The listing builds one solid part. Answer for the finished solid, in the listing's coordinates (mm). Face numbers are marked on the shaded views. A direction names the side the tool comes from. Give positions to 0.01 mm unless a question says otherwise; leave off trailing zeros. Order: outer loops, then holes, each group sorted by start corner. A loop starts at its lowest first (then second) coordinate and runs counter-clockwise, first axis right, second up. Notation, with made-up numbers: (87.5, -12) - (114.5, -12) arc R14 cw to (114.5, 10) - close; hole circle Ø7 at (-32.75, 1). An arc over 180 degrees is marked (long way). Answer as CSV lines item,"result". Start each with the question number.
1. Section A-A on z = 1.5 is taken. Give the vertices of the cut face in (x, y) (3 decimals), and give its area (3 significant figures).
2. Which of the six approach directions +Z, -Z, +X, -X, +Y, -Y give full straight-line access (tool end or side, diameter ignored) to the marked faces 1, 2 and 3?
3. Section C-C on y = -13.9 is taken. Give the vertices of the cut face in (x, z) (3 decimals), and give its area (3 significant figures).
4. Determine the mould class of the marked faces 4, 5 and 6 for opening direction Z: +Z half, -Z half, draft (parallel to the pull), parting line (faces both ways), or undercut.
5. Section D-D on z = -1.25 is taken. Give the vertices of the cut face in (x, y) (3 decimals).
6. Flat-ended cylindrical pins translate along their axes: pin 1 (0.6 mm diameter, centred on x = -8.5, z = -7.5, fed in from +Y); pin 2 (1.6 mm diameter, centred on x = -9, y = 1, fed in from -Z); pin 3 (1.6 mm diameter, centred on x = 0, y = -13.9, fed in from +Z); pin 4 (4 mm diameter, centred on x = 0, y = 13.9, fed in from -Z). Find the tip coordinate at first contact, or state that the pin passes through.
7. Section B-B on x = 4 is taken. Give the vertices of the cut face in (y, z), and give its area (3 significant figures).
8. Consider line 1 along Y through (x, z) = (0, 4.3); line 2 along Z through (x, y) = (-4.15, -12.1) (3 decimals); line 3 along Y through (x, z) = (0, -3.25). Determine where each line is inside the solid, lowest interval first. Write a range as [from, to].
Autodesk Inventor part; units mm, degrees
ref_plane "Work Plane1" through (-1.325, -11.4, 0) normal (-1, 0, 0) x (0, 0, 1)
ref_plane "Work Plane3" through (0, -16.6, 5) normal (-1, 0, 0) x (0, 0, 1)
ref_plane "YZ Plane" through (0, 0, 0) normal (1, 0, 0) x (0, 1, 0)
sketch "Sketch1" plane through (0, 0, 0) normal (0, 0, 1) x (1, 0, 0)
  line L0 (-9.975, 16.6) -> (9.975, 16.6)
  line L1 (9.975, 16.6) -> (9.975, -16.6)
  line L2 (9.975, -16.6) -> (-9.975, -16.6)
  line L3 (-9.975, -16.6) -> (-9.975, 16.6)
  line L4 (0, 0) -> (0, 11.4) construction
  line L5 (0, 0) -> (15.5803, 0) construction
  line L6 (-6.15, 11.4) -> (6.15, 11.4)
  line L7 (6.15, 11.4) -> (6.15, -11.4)
  line L8 (6.15, -11.4) -> (-6.15, -11.4)
  line L9 (-6.15, -11.4) -> (-6.15, 11.4)
  circle A0 centre (0, 13.9) radius 1.3
  circle A1 centre (0, -13.9) radius 1.3
  line L10 (-15.0861, 0) -> (20.6914, 0)
  line L11 (9.975, -16.6) -> (-9.975, -16.6)
  line L12 (-9.975, -16.6) -> (-9.975, -11.4)
  line L13 (-9.975, -11.4) -> (9.975, -11.4)
  line L14 (9.975, -11.4) -> (9.975, -16.6)
  line L15 (0, 11.4) -> (0, 13.9) construction
  point P0 (0, 16.6)
  dimension "d0" = 2.6
  dimension "d1" = 27.8
  dimension "d4" = 12.3
  dimension "d5" = 2.5
  dimension "d6" = 2.5
  dimension "d7" = 22.8
  dimension "d11" = 2.7
  dimension "d12" = 2.7
  dimension "d14" = 3.825
extrude "Extrusion1" add sketch "Sketch1" along normal blind 5 contours L0 L1 L10 L7 L6 L9 L3 | L10 L9 L13 L3 | L1 L13 L7 L10 | L13 L8 L1 L2 L3
extrude "Extrusion2" add sketch "Sketch1" against normal blind 15.8 contours L13 L8 L1 L2 L3
sketch "Sketch2" plane through (-6.15, -11.4, 5) normal (0, 1, 0) x (1, 0, 0)
  circle A0 centre (10.3, 15.485) radius 1.05
  circle A1 centre (2, 15.485) radius 1.05
  line L0 (-3.825, 20.8) -> (16.125, 20.8)
  line L1 (-3.825, 5) -> (-3.825, 20.8)
  line L2 (2, 15.485) -> (10.3, 15.485) construction
  line L3 (10.3, 15.485) -> (6.15, 15.485) construction
  line L4 (6.15, 15.485) -> (6.15, 20.8) construction
  point P0 (6.15, 5)
  dimension "d19" = 2.1
  dimension "d20" = 0
  dimension "d21" = 5.315
  dimension "d22" = 8.3
extrude "Extrusion3" cut sketch "Sketch2" against normal blind 10
sketch "Sketch3" plane through (-6.15, -11.4, 5) normal (0, 1, 0) x (1, 0, 0)
  circle A0 centre (10.3, 15.485) radius 1.05
  circle A1 centre (10.3, 15.485) radius 2.5
  circle A2 centre (2, 15.485) radius 1.05
  circle A3 centre (2, 15.485) radius 2.5
  point P0 (6.15, 5)
  dimension "d26" = 5
extrude "Extrusion4" cut sketch "Sketch3" against normal blind 2
sketch "Sketch4" plane through (9.975, -11.4, 0) normal (1, 0, 0) x (0, 0, -1)
  line L0 (0, 0) -> (15.8, 0)
  line L1 (0, 0) -> (0, 28)
  line L2 (15.8, 0) -> (0, 28)
  line L3 (0, 28) -> (0, 11.7214)
  line L4 (0, 11.7214) -> (6.6142, 0)
  line L5 (6.6142, 0) -> (15.8, 0)
  line L6 (0, 28) -> (-5, 28)
  line L7 (0, 11.7214) -> (0, 28)
  line L8 (6, 17.3671) -> (11.2857, 17.3671)
  line L9 (11.2857, 17.3671) -> (11.2857, 8)
  line L10 (11.2857, 8) -> (6, 8)
  line L11 (6, 8) -> (6, 17.3671)
  point P0 (0, 11.4)
  dimension "d29" = 8
  dimension "d33" = 8
  dimension "d34" = 6
ref_plane "Work Plane1" through (-1.325, -11.4, 0) normal (-1, 0, 0) x (0, 0, 1)
extrude "Extrusion5" add sketch "Sketch4" against normal blind 2 contours L4 L1 L2 L11 L10 L0
ref_plane "Work Plane3" through (0, -16.6, 5) normal (-1, 0, 0) x (0, 0, 1)
mirror "Mirror1" about plane through (0, -16.6, 5) normal (-1, 0, 0) of "Extrusion5"
fillet "Fillet1" radius 2 6 edges at (8.975, 0.3214, 0) (8.975, -11.4, -6.6142) (8.0625, -11.4, 0) (-8.975, -11.4, -6.6142) (-8.0625, -11.4, 0) (-8.975, 0.3214, 0)
sketch "Sketch5" plane through (-9.975, -16.6, 5) normal (0, -1, 0) x (1, 0, 0)
  line L0 (0, 0) -> (19.95, 0)
  line L1 (7.875, -3) -> (12.075, -3)
  line L2 (12.075, -3) -> (12.075, -5)
  line L3 (12.075, -5) -> (7.875, -5)
  line L4 (7.875, -5) -> (7.875, -3)
  line L5 (9.975, 0) -> (9.975, -3) construction
  point P0 (9.975, -5)
  dimension "d39" = 4.2
  dimension "d40" = 3
  dimension "d41" = 2
extrude "Extrusion7" cut sketch "Sketch5" against normal through all
properties part number "GrabberServoHolder_3DPrint"
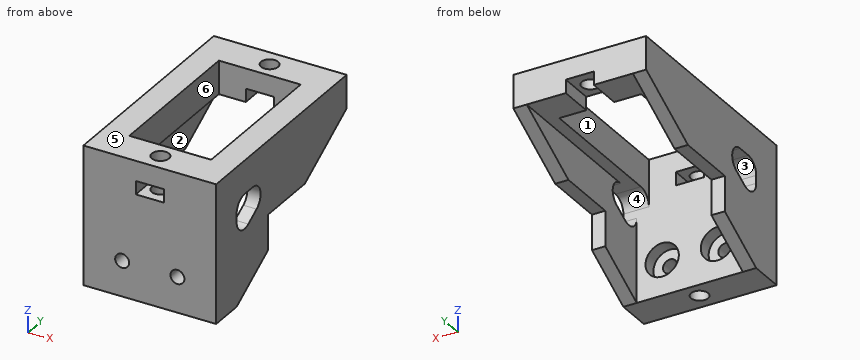
Checks:
1,outline,"(-9.975, -16.6) - (-2.1, -16.6) - (-2.1, -11.4) - (-6.15, -11.4) - (-6.15, 11.4) - (-2.1, 11.4) - (-2.1, 16.6) - (-9.975, 16.6) - close; (2.1, -16.6) - (9.975, -16.6) - (9.975, 16.6) - (2.1, 16.6) - (2.1, 11.4) - (6.15, 11.4) - (6.15, -11.4) - (2.1, -11.4) - close"
1,area,"338 mm²"
2,face 1,"+Z, -Z"
2,face 2,"-Z, +Y"
2,face 3,"+X, -X"
3,outline,"(-9.975, -15.8) - (-1.3, -15.8) - (-1.3, 0) - (-2.1, 0) - (-2.1, 2) - (-1.3, 2) - (-1.3, 5) - (-9.975, 5) - close; (1.3, -15.8) - (9.975, -15.8) - (9.975, 5) - (1.3, 5) - (1.3, 2) - (2.1, 2) - (2.1, 0) - (1.3, 0) - close; hole circle Ø2.1 at (-4.15, -10.485); hole circle Ø2.1 at (4.15, -10.485)"
3,area,"351 mm²"
4,face 4,"undercut"
4,face 5,"+Z half"
4,face 6,"draft"
5,outline,"(-9.975, -16.6) - (9.975, -16.6) - (9.975, -11.254) - (6.15, -11.254) - (6.15, -11.4) - (-6.15, -11.4) - (-6.15, -11.254) - (-9.975, -11.254) - close; (-9.975, -5.439) - (-7.975, -5.439) - (-7.975, 14.385) - (-9.975, 14.385) - close; (7.975, -5.439) - (9.975, -5.439) - (9.975, 14.385) - (7.975, 14.385) - close; hole circle Ø2.6 at (0, -13.9)"
6,pin 1,"stops at y = -3.4"
6,pin 2,"stops at z = -6"
6,pin 3,"passes through"
6,pin 4,"stops at z = 2"
7,outline,"(-16.6, -15.8) - (-11.4, -15.8) - (-11.4, -12.98) - (-13.4, -12.98) - (-13.4, -11.52) - (-16.6, -11.52) - close; (-16.6, -9.45) - (-13.4, -9.45) - (-13.4, -7.99) - (-11.4, -7.99) - (-11.4, 5) - (-16.6, 5) - close; (11.4, 0) - (16.6, 0) - (16.6, 5) - (11.4, 5) - close"
7,area,"118 mm²"
8,line 1,"y = [-16.6, -15.2], [-12.6, -11.4], [11.4, 12.6], [15.2, 16.6]"
8,line 2,"z = [-15.8, -12.985], [-7.985, 5]"
8,line 3,"y = [-16.6, -15.2], [-12.6, -11.4]"
